Design review of the part built by this model. Coordinates are the model's own, in mm. Round coordinates to 2 decimals unless told otherwise and drop trailing zeros. Write each loop counter-clockwise with the first axis right and the second up, starting at its lowest first coordinate (ties: lowest second). Pieces come first, ordered by that corner, then holes. Notation, with made-up numbers: M -13,24.25 L 17,24.25 A9 ccw 17,29.25 Z; hole C 87.5,-38.5 d7. An arc over 180 degrees is marked long. One line per question, with ' | ' between items. Start each with the question number.
Item 1: Insertion check: pin 1 Ø0.9 at (y, z) = (1, 10) entering from +X. The pin has a flat end and moves straight along its axis. Give the tip position at first contact, or say it passes through.
Item 2: Add section A-A, the plane z = 1. State the section outline as (x, y) points.
Item 3: For L1, parallel to X at y = 1.25, z = 11; L2, parallel to Z at x = 85, y = 1.2; L3, parallel to X at y = 0.8, z = 28, list the stretches that pass through material, from the lowest coordinate up.
Item 4: Add section D-D, the plane y = 2.5. State the section outline as (x, z) points (1 decimal), and give its area (3 significant figures).
Item 5: Add section B-B, the plane x = 16.5. State the section outline as (y, z) points.
Item 6: Add section C-C, the plane z = 30. State the section outline as (x, y) points, and give its area (3 significant figures).
```python
from build123d import *

# Parameters (mm, degrees)
ESQUISSE1_R             = 2.5
BOSS_EXTRU_1_DEPTH      = 3
ENL_V_MAT_EXTRU_1_DEPTH = 166.064843505


with BuildPart() as part:
    # Esquisse1 → Boss.-Extru.1 (new body)
    with BuildSketch(Plane(origin=(0, 0, 0), x_dir=(1, 0, 0), z_dir=(0, 1, 0))):
        Polygon((-161.174292495, 18.77), (-161.174292495, -25.5), (-161.174292495, -35.5), (138.625707505, -35.5), (138.625707505, -10.5), (73.911950915, -10.5), (73.911950915, 28.77), (-161.174292495, 28.77), align=None)
        with Locations(Location((-151.374292495, -19.4325, 0), (0, 0, 270))):
            Circle(ESQUISSE1_R, mode=Mode.SUBTRACT)
        with Locations(Location((-151.374292495, 12.7025, 0), (0, 0, 270))):
            Circle(ESQUISSE1_R, mode=Mode.SUBTRACT)
        with Locations(Location((53.861950915, 10.635, 0), (0, 0, 270))):
            Circle(ESQUISSE1_R, mode=Mode.SUBTRACT)
        Polygon((114.261515644, -15.687745544), (114.261515644, -18.634239014), (132.625707505, -18.634239014), (132.625707505, -32.887044638), (114.261515644, -32.887044638), (79.109163313, -32.887044638), (79.109163313, -15.687745544), align=None, mode=Mode.SUBTRACT)
    extrude(amount=BOSS_EXTRU_1_DEPTH)

    # Esquisse2 → Enlèv. mat.-Extru.1 (cut, through all)
    with BuildSketch(Plane.XZ):
        with BuildLine():
            Line((7.640390062, -11.635), (7.640390062, 18.365))
            ThreePointArc((7.640390062, 18.365), (15.140390062, 25.865), (22.640390062, 18.365))
            Line((22.640390062, 18.365), (22.640390062, -11.635))
            ThreePointArc((22.640390062, -11.635), (15.140390062, -19.135), (7.640390062, -11.635))
        make_face()
        with BuildLine():
            Line((-51.13117079, -11.635), (-51.13117079, 18.365))
            ThreePointArc((-51.13117079, 18.365), (-43.63117079, 25.865), (-36.13117079, 18.365))
            Line((-36.13117079, 18.365), (-36.13117079, -11.635))
            ThreePointArc((-36.13117079, -11.635), (-43.63117079, -19.135), (-51.13117079, -11.635))
        make_face()
        with BuildLine():
            Line((-109.902731643, -11.635), (-109.902731643, 18.365))
            ThreePointArc((-109.902731643, 18.365), (-102.402731643, 25.865), (-94.902731643, 18.365))
            Line((-94.902731643, 18.365), (-94.902731643, -11.635))
            ThreePointArc((-94.902731643, -11.635), (-102.402731643, -19.135), (-109.902731643, -11.635))
        make_face()
    extrude(amount=-ENL_V_MAT_EXTRU_1_DEPTH, mode=Mode.SUBTRACT)


solid = part.part
```
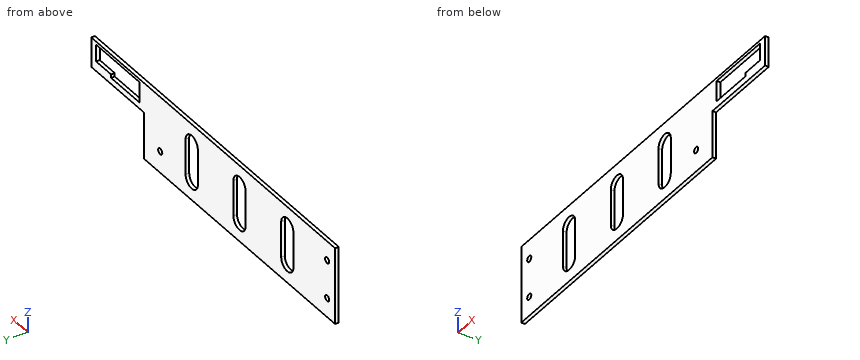
Computed values:
1) pin 1: stops at x = 73.91
2) outline: M -161.17,0 L -109.9,0 L -109.9,3 L -161.17,3 Z; M -94.9,0 L -51.13,0 L -51.13,3 L -94.9,3 Z; M -36.13,0 L 7.64,0 L 7.64,3 L -36.13,3 Z; M 22.64,0 L 73.91,0 L 73.91,3 L 22.64,3 Z
3) L1: x = -161.17 to -109.9, -94.9 to -51.13, -36.13 to 7.64, 22.64 to 138.63 | L2: z = 10.5 to 15.69, 32.89 to 35.5 | L3: x = -161.17 to 79.11, 132.63 to 138.63
4) outline: M -161.2,-28.8 L 73.9,-28.8 L 73.9,10.5 L 138.6,10.5 L 138.6,35.5 L -161.2,35.5 Z; hole C -151.4,-12.7 d5; hole C -151.4,19.4 d5; hole M -109.9,-11.6 A7.5 ccw -94.9,-11.6 L -94.9,18.4 A7.5 ccw -109.9,18.4 Z; hole M -51.1,-11.6 A7.5 ccw -36.1,-11.6 L -36.1,18.4 A7.5 ccw -51.1,18.4 Z; hole M 7.6,-11.6 A7.5 ccw 22.6,-11.6 L 22.6,18.4 A7.5 ccw 7.6,18.4 Z; hole C 53.9,-10.6 d5; hole M 79.1,15.7 L 114.3,15.7 L 114.3,18.6 L 132.6,18.6 L 132.6,32.9 L 79.1,32.9 Z | area: 13,900 mm^2
5) outline: M 0,-28.77 L 3,-28.77 L 3,-19.01 L 0,-19.01 Z; M 0,25.74 L 3,25.74 L 3,35.5 L 0,35.5 Z
6) outline: M -161.17,0 L 79.11,0 L 79.11,3 L -161.17,3 Z; M 132.63,0 L 138.63,0 L 138.63,3 L 132.63,3 Z | area: 739 mm^2
